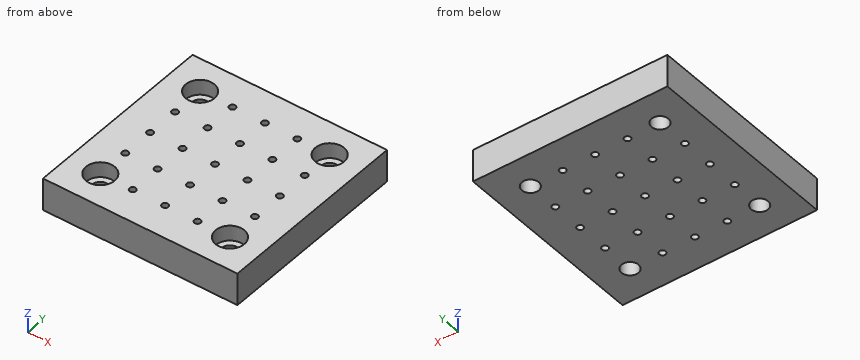
```python
from build123d import *

# Parameters (mm, degrees)
F0_W           = 76.2
F0_H           = 76.2
F1_DEPTH       = 12.7
F2_D           = 2.5
F3_D           = 6.6
F3_CBORE_D     = 11.25
F3_CBORE_DEPTH = 6


with BuildPart() as f1:
    # F0 (on Top) → F1 (new body)
    with BuildSketch(Plane.XY):
        Rectangle(F0_W, F0_H)
    extrude(amount=-F1_DEPTH)

    # F2 (through all)
    with Locations(Plane.XY):
        with Locations((-25.4, 12.7), (-12.7, 25.4), (-12.7, 12.7), (0, 12.7), (12.7, 25.4), (0, 25.4), (12.7, 12.7), (25.4, 12.7), (25.4, 0), (12.7, 0), (0, 0), (-12.7, 0), (-25.4, 0), (-25.4, -12.7), (-12.7, -12.7), (0, -12.7), (12.7, -12.7), (25.4, -12.7), (12.7, -25.4), (0, -25.4), (-12.7, -25.4)):
            Hole(F2_D / 2)

    # F3 (through all)
    with Locations(Plane.XY):
        with Locations((-25.4, 25.4), (25.4, 25.4), (25.4, -25.4), (-25.4, -25.4)):
            CounterBoreHole(F3_D / 2, F3_CBORE_D / 2, F3_CBORE_DEPTH)


solid = f1.part
```
Input: part model. Units: mm. Frame: model coordinates. Coordinates: 2 decimals unless noted, no trailing zeros. Loops run counter-clockwise (first coordinate to the right, second up) from the corner with the lowest first, then second, coordinate; pieces in that order, holes last. Notation, with made-up numbers: M -14,19 L 9,19 A22 cw 9,30 Z; hole C -29,-38.5 d3. An arc over 180 degrees is marked long. One line per item, written item: value.
(1) Pin query (flat end, axial travel): pin 1 (2 mm diameter, centred on x = 0, y = 25.4, fed in from +Z); pin 2 (10 mm diameter, centred on x = 25.4, y = 25.4, fed in from +Z). Return the tip coordinate at first contact, or that it passes through.
Filled in:
pin 1: through
pin 2: z = -6
(2) Section A-A (x = 0). Output: boundary loops of the cut face in (y, z).
Filled in:
outline: M -38.1,-12.7 L -26.65,-12.7 L -26.65,0 L -38.1,0 Z; M -24.15,-12.7 L -13.95,-12.7 L -13.95,0 L -24.15,0 Z; M -11.45,-12.7 L -1.25,-12.7 L -1.25,0 L -11.45,0 Z; M 1.25,-12.7 L 11.45,-12.7 L 11.45,0 L 1.25,0 Z; M 13.95,-12.7 L 24.15,-12.7 L 24.15,0 L 13.95,0 Z; M 26.65,-12.7 L 38.1,-12.7 L 38.1,0 L 26.65,0 Z
(3) Section B-B (z = -3). Give the number of separate pieces and of enclosed holes in the cut face, and give its area (3 significant figures).
Filled in:
separate pieces: 1
enclosed holes: 25
area: 5,310 mm^2
(4) Line query: line 1 along Y through (x, z) = (-25.4, -8.5); line 2 along Y through (x, z) = (-25.4, -1.45) (3 decimals); line 3 along X through (y, z) = (-22, -2). Output: solid intervals per line, ascending. Write a range as from..to.
Filled in:
line 1: -38.1..-28.7, -22.1..-13.95, -11.45..-1.25, 1.25..11.45, 13.95..22.1, 28.7..38.1
line 2: -38.1..-31.025, -19.775..-13.95, -11.45..-1.25, 1.25..11.45, 13.95..19.775, 31.025..38.1
line 3: -38.1..-29.88, -20.92..20.92, 29.88..38.1
